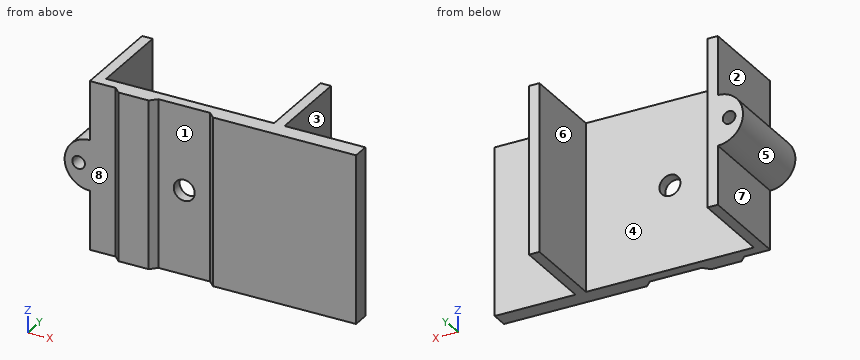
from build123d import *

# Parameters (mm, degrees)
BOSS_EXTRUDE2_DEPTH             = 80
SKETCH2_R                       = 3
BOSS_EXTRUDE3_DEPTH             = 45
SKETCH3_R                       = 5
CUT_EXTRUDE1_DEPTH              = 8.959911114
BOSS_EXTRUDE4_DEPTH             = 38.5
BOSS_EXTRUDE4_DIRECTION_2_REACH = 104


with BuildPart() as part:
    # Sketch1 → Boss-Extrude2 (new body)
    with BuildSketch(Plane.XY):
        Polygon((9.382877742, 0), (0, 0), (0, 40), (-5, 40), (-5, -5), (7.31180993, -5), (10.271721045, -7.959911114), (24.701165041, -7.959911114), (27.661076156, -5), (52.338923844, -5), (55.298834959, -7.959911114), (69.728278955, -7.959911114), (72.68819007, -5), (85, -5), (85, 40), (80, 40), (80, 0), (70.617122258, 0), (54.409991656, 0), (25.590008344, 0), align=None)
    extrude(amount=BOSS_EXTRUDE2_DEPTH)

    # Sketch2 → Boss-Extrude3 (add)
    with BuildSketch(Plane(origin=(0, 40, 0), x_dir=(1, 0, 0), z_dir=(0, 1, 0))):
        with BuildLine():
            Line((-5, -28), (-5, -52))
            ThreePointArc((-5, -52), (-17, -40), (-5, -28))
        make_face()
        with Locations((-10.338111961, -40)):
            Circle(SKETCH2_R, mode=Mode.SUBTRACT)
    extrude(amount=-BOSS_EXTRUDE3_DEPTH)

    # Sketch3 → Cut-Extrude1 (cut, through all)
    with BuildSketch(Plane(origin=(0, 0, 0), x_dir=(1, 0, 0), z_dir=(0, 1, 0))):
        with Locations((40, -40)):
            Circle(SKETCH3_R)
    extrude(amount=-CUT_EXTRUDE1_DEPTH, mode=Mode.SUBTRACT)

    # Sketch5 → Boss-Extrude4 (add)
    with BuildSketch(Plane(origin=(85, 0, 0), x_dir=(0, 0, -1), z_dir=(1, 0, 0))):
        Polygon((-80, -5), (-80, -7.959911114), (0, -7.959911114), (0, -5), (0, 0), (-80, 0), align=None)
    extrude(amount=BOSS_EXTRUDE4_DEPTH)

    # Boss-Extrude4 direction 2: up to this face of the body (flat: up to its plane)
    boss_extrude4_direction_2_end = Plane(part.part.faces().sort_by_distance((71.208234512, -6.479955557, 40))[0])
    # Sketch5 → Boss-Extrude4 direction 2 (add, up to the picked face)
    with BuildSketch(Plane(origin=(85, 0, 0), x_dir=(0, 0, -1), z_dir=(1, 0, 0)), mode=Mode.PRIVATE) as boss_extrude4_direction_2_sk1:
        Polygon((-80, -5), (-80, -7.959911114), (0, -7.959911114), (0, -5), (0, 0), (-80, 0), align=None)
    boss_extrude4_direction_2_tool1 = split(extrude(boss_extrude4_direction_2_sk1.sketch, amount=-BOSS_EXTRUDE4_DIRECTION_2_REACH, mode=Mode.PRIVATE), bisect_by=boss_extrude4_direction_2_end, keep=Keep.BOTH, mode=Mode.PRIVATE)
    add(boss_extrude4_direction_2_tool1.solids().sort_by_distance((85, -3.979956, 40))[0])


solid = part.part
Work out the finished part from the listing and answer in its coordinate system (mm). Face numbers are marked on the shaded views. A direction names the side the tool comes from. Round coordinates to 2 decimals unless told otherwise and drop trailing zeros. Loops run counter-clockwise (first coordinate to the right, second up) from the corner with the lowest first, then second, coordinate; pieces in that order, holes last. Notation, with made-up numbers: (24, 60) - (48, 60) arc R8 cw to (48, 66) - close; hole circle Ø8 at (53, 73.5). An arc over 180 degrees is marked (long way). One line per item, written item: value.
Q1. For the marked faces 1, 2, 3, 4 and 5, determine the directions among +Z, -Z, +X, -X, +Y, -Y from which every point of the face is accessible in a straight line to the end or side of a thin tool.
Check values:
face 1: +Z, -Z, -Y
face 2: +Z, -X, +Y, -Y
face 3: +Z, -Z, +X, +Y
face 4: +Z, -Z, +Y
face 5: -X, +Y, -Y
Q2. Find section B-B on x = 40. Give the vertices of the cut face in (y, z), and give its area (3 significant figures).
Check values:
outline: (-5, 0) - (0, 0) - (0, 35) - (-5, 35) - close; (-5, 45) - (0, 45) - (0, 80) - (-5, 80) - close
area: 350 mm2
Q3. Find section A-A on y = 9.5. Give the vertices of the cut face in (x, z), and give its area (3 significant figures).
Check values:
outline: (-5, 0) - (0, 0) - (0, 80) - (-5, 80) - (-5, 52) arc R12 ccw to (-5, 28) - close; (80, 0) - (85, 0) - (85, 80) - (80, 80) - close; hole circle Ø6 at (-10.34, 40)
area: 998 mm2
Q4. Find section D-D on y = -3.5. Give the vertices of the cut face in (x, z), and give its area (3 significant figures).
Check values:
outline: (-5, 0) - (123.5, 0) - (123.5, 80) - (-5, 80) - (-5, 52) arc R12 ccw to (-5, 28) - close; hole circle Ø6 at (-10.34, 40); hole circle Ø10 at (40, 40)
area: 10,400 mm2
Q5. Each of these flat-tipped pins is pushed along its axis until it touches: pin 1 Ø10 at (x, y) = (106.5, 6) entering from -Z; pin 2 Ø19.5 at (x, z) = (-5.5, 33) entering from -Y; pin 3 Ø8.5 at (y, z) = (26, 15) entering from -X; pin 4 Ø20 at (y, z) = (16.5, 52.5) entering from -X. Where does it stop, or does it pass through?
Check values:
pin 1: through
pin 2: y = -5
pin 3: x = -5
pin 4: x = -16.74
Q6. The mould has two halves that part along X. Classify the marked faces 6, 7 and 8: +X half, -X half, draft (parallel to the pull), parting line (faces both ways), or undercut.
Check values:
face 6: undercut
face 7: -X half
face 8: draft
Q7. Straight lines are drawn through the part: probe 1 along X at (y, z) = (10, 40); probe 2 along X at (y, z) = (-1.85, 40); probe 3 along X at (y, z) = (4.5, 11). For each, find the intervals that lie inside material, in ascending order.
Check values:
probe 1: -17 to -13.34, -7.34 to 0, 80 to 85
probe 2: -17 to -13.34, -7.34 to 35, 45 to 123.5
probe 3: -5 to 0, 80 to 85
Q8. Find section C-C on z = 40. Give the vertices of the cut face in (x, y), and give its area (3 significant figures).
Check values:
outline: (-17, -5) - (-13.34, -5) - (-13.34, 40) - (-17, 40) - close; (-7.34, -5) - (7.31, -5) - (10.27, -7.96) - (24.7, -7.96) - (27.66, -5) - (35, -5) - (35, 0) - (0, 0) - (0, 40) - (-7.34, 40) - close; (45, -5) - (52.34, -5) - (55.3, -7.96) - (123.5, -7.96) - (123.5, 0) - (85, 0) - (85, 40) - (80, 40) - (80, 0) - (45, 0) - close
area: 1,520 mm2
